Could you check a few things on this model? Use its own coordinates, in mm. A direction names the side the tool comes from. Give positions to 0.01 mm unless a question says otherwise; leave off trailing zeros. Loops run counter-clockwise (first coordinate to the right, second up) from the corner with the lowest first, then second, coordinate; pieces in that order, holes last. Notation, with made-up numbers: (87, 82.25) -> (116, 82.25) arc R16 cw to (116, 92.25) -> close; hole circle Ø11 at (-40, 84). An arc over 180 degrees is marked (long way). Write item = value, one per line. Start each with the question number.
1) On a 3-axis mill with a long thin cutter (end or side, diameter ignored), from which of +Z, -Z, +X, -X, +Y, -Y can I reach the whole of each face in a straight line? I mean faces 1 (the face through (-10, 10, 0)), 2 (the face through (-5, -8.8, -9.9)), 3 (the face through (-9.15, -4.01, -8.95)). Say none if no direction works.
2) I want a section at C-C (z = 12.5). Count the separate pieces of the cut face and the enclosed holes in it, and give its area (3 significant figures).
3) If we mould it in two halves opening along X, with no side actions, what happens to faces 4 (the face through (12, 0, 11)), 5 (the face through (-10, -10, 1)), 6 (the face through (15, -11, 11))? For each: +X half, -X half, draft (parallel to the pull), parting line (faces both ways), or undercut.
4) I want a section at D-D (y = 16). List the corners of the cut face in (x, z) for me.
5) I'm going to push flat-ended pins straight in: pin 1 Ø3 at (y, z) = (-5, 2) entering from -X; pin 2 Ø5.5 at (x, y) = (-12, 10.5) entering from +Z; pin 3 Ø6 at (x, z) = (-4.5, -10) entering from -Y. Where does each tip first touch, or does it pass through?
6) I want a section at A-A (x = 10). List the corners of the cut face in (y, z) for me, and give its area (3 significant figures).
7) I need wall thicknesses on probe 1 along Y at (x, z) = (10, 4.3); probe 2 along Z at (x, y) = (-4.1, -12.5); probe 3 along Z at (x, y) = (10, -0.95). Which ranges of each line are inside material? Lowest first, please. Write a range as from..to.
from build123d import *

# Parameters (mm, degrees)
F1_DEPTH  = 5
F3_DEPTH  = 20
F5_DEPTH  = 40.001
F7_DEPTH  = 40.001
F8_R      = 2.01
F9_DEPTH  = 5
F10_R     = 2.01
F11_DEPTH = 5
F12_R     = 3.51
F13_DEPTH = 2
F14_R     = 3.51
F15_DEPTH = 2
F16_R     = 2.01
F17_DEPTH = 5
F18_R     = 3.51
F19_DEPTH = 2
F20_R     = 3.51
F21_DEPTH = 2
F23_DEPTH = 20
F24_R     = 2.01
F25_DEPTH = 5
F26_R     = 2.01
F27_DEPTH = 5
F28_R     = 3.51
F29_DEPTH = 2
F30_R     = 3.51
F31_DEPTH = 2
F32_W     = 20
F32_H     = 2
F33_DEPTH = 20.001
F35_DEPTH = 20.001


with BuildPart() as f1:
    # F0 (on Top) → F1 (new body)
    with BuildSketch(Plane.XY):
        Polygon((20, 0), (0, 0), (0, 20), (-20, 20), (-20, 0), (0, -20), (20, -20), align=None)
    extrude(amount=F1_DEPTH)

    # F2 (on face) → F3 (join)
    with BuildSketch(Plane.XY.offset(5)):
        Polygon((15, -20), (20, -20), (20, 0), (0, 0), (0, 20), (-5, 20), (-20, 20), (-20, 15), (-5, 15), (-5, 5), (-20, 5), (-20, 0), (-5, 0), (0, -5), (0, -20), (5, -20), (5, -5), (15, -5), align=None)
    extrude(amount=F3_DEPTH)

    # F4 (on face) → F5 (cut, through all)
    with BuildSketch(Plane.YZ.offset(20)):
        Polygon((-20, 5), (0, 25), (-20, 25), align=None)
    extrude(amount=-F5_DEPTH, mode=Mode.SUBTRACT)

    # F6 (on face) → F7 (cut, through all)
    with BuildSketch(Plane(origin=(0, 20, 0), x_dir=(-1, 0, 0), z_dir=(0, 1, 0))):
        Polygon((0, 25), (20, 5), (20, 25), align=None)
    extrude(amount=-F7_DEPTH, mode=Mode.SUBTRACT)

    # F8 (on face) → F9 (cut)
    with BuildSketch(Plane.YZ):
        with Locations((10, 12.5)):
            Circle(F8_R)
    extrude(amount=-F9_DEPTH, mode=Mode.SUBTRACT)

    # F10 (on face) → F11 (cut)
    with BuildSketch(Plane(origin=(0, 0, 0), x_dir=(-1, 0, 0), z_dir=(0, 1, 0))):
        with Locations((-10, 12.5)):
            Circle(F10_R)
    extrude(amount=-F11_DEPTH, mode=Mode.SUBTRACT)

    # F12 (on face) → F13 (cut)
    with BuildSketch(Plane.XZ.offset(5)):
        with Locations((10, 12.5)):
            Circle(F12_R)
    extrude(amount=-F13_DEPTH, mode=Mode.SUBTRACT)

    # F14 (on face) → F15 (cut)
    with BuildSketch(Plane(origin=(-5, 0, 0), x_dir=(0, -1, 0), z_dir=(-1, 0, 0))):
        with Locations((-10, 12.5)):
            Circle(F14_R)
    extrude(amount=-F15_DEPTH, mode=Mode.SUBTRACT)

    # F16 (on face) → F17 (cut)
    with BuildSketch(Plane(origin=(0, 0, 0), x_dir=(1, 0, 0), z_dir=(0, 0, -1))):
        with Locations((-12.5, -10)):
            Circle(F16_R)
        with Locations((10, 12.5)):
            Circle(F16_R)
    extrude(amount=-F17_DEPTH, mode=Mode.SUBTRACT)

    # F18 (on face) → F19 (cut)
    with BuildSketch(Plane.XY.offset(5)):
        with Locations((-12.5, 10)):
            Circle(F18_R)
    extrude(amount=-F19_DEPTH, mode=Mode.SUBTRACT)

    # F20 (on face) → F21 (cut)
    with BuildSketch(Plane.XY.offset(5)):
        with Locations((10, -12.5)):
            Circle(F20_R)
    extrude(amount=-F21_DEPTH, mode=Mode.SUBTRACT)

    # F22 (on Top) → F23 (join)
    with BuildSketch(Plane.XY):
        Polygon((0, -20), (0, 0), (-20, 0), (-15, -5), (-10, -5), (-5, -5), (-5, -10), (-5, -15), align=None)
    extrude(amount=-F23_DEPTH)

    # F24 (on face) → F25 (cut)
    with BuildSketch(Plane.YZ):
        with Locations((-12.5, -10)):
            Circle(F24_R)
    extrude(amount=-F25_DEPTH, mode=Mode.SUBTRACT)

    # F26 (on face) → F27 (cut)
    with BuildSketch(Plane(origin=(0, 0, 0), x_dir=(-1, 0, 0), z_dir=(0, 1, 0))):
        with Locations((12.5, -10)):
            Circle(F26_R)
    extrude(amount=-F27_DEPTH, mode=Mode.SUBTRACT)

    # F28 (on face) → F29 (cut)
    with BuildSketch(Plane(origin=(-5, 0, 0), x_dir=(0, -1, 0), z_dir=(-1, 0, 0))):
        with Locations((12.5, -10)):
            Circle(F28_R)
    extrude(amount=-F29_DEPTH, mode=Mode.SUBTRACT)

    # F30 (on face) → F31 (cut)
    with BuildSketch(Plane.XZ.offset(5)):
        with Locations((-12.5, -10)):
            Circle(F30_R)
    extrude(amount=-F31_DEPTH, mode=Mode.SUBTRACT)

    # F32 (on face) → F33 (cut, through all)
    with BuildSketch(Plane(origin=(0, 0, 0), x_dir=(-1, 0, 0), z_dir=(0, 1, 0))):
        with Locations((-10, 24)):
            Rectangle(F32_W, F32_H)
    extrude(amount=-F33_DEPTH, mode=Mode.SUBTRACT)

    # F34 (on face) → F35 (cut, through all)
    with BuildSketch(Plane.YZ):
        Polygon((-2.924178, 22.901505), (-2, 23), (20, 23), (20, 25), (-2.924178, 25), align=None)
    extrude(amount=-F35_DEPTH, mode=Mode.SUBTRACT)


solid = f1.part
Answer list:
q1.face_1 = -Z, +X, -X, +Y
q1.face_2 = -Z, -X, -Y
q1.face_3 = -Y
q2.separate_pieces = 3
q2.enclosed_holes = 0
q2.area = 310 mm^2
q3.face_4 = draft
q3.face_5 = -X half
q3.face_6 = undercut
q4.outline = (-20, 0) -> (0, 0) -> (0, 23) -> (-2, 23) -> (-20, 5) -> close
q5.pin_1 = -16.5
q5.pin_2 = 3
q5.pin_3 = -18.5
q6.outline = (-20, 0) -> (-14.51, 0) -> (-14.51, 3) -> (-16.01, 3) -> (-16.01, 5) -> (-20, 5) -> close; (-10.49, 0) -> (0, 0) -> (0, 10.49) -> (-3, 10.49) -> (-3, 8.99) -> (-5, 8.99) -> (-5, 5) -> (-8.99, 5) -> (-8.99, 3) -> (-10.49, 3) -> close; (-5, 16.01) -> (-3, 16.01) -> (-3, 14.51) -> (0, 14.51) -> (0, 23) -> (-2, 23) -> (-5, 20) -> close
q6.area = 133 mm^2
q7.probe_1 = -20..-16.01, -8.99..0
q7.probe_2 = -20..-13.51, -6.49..5
q7.probe_3 = 0..10.49, 14.51..23
